Design review of the part shown in the three views and the two pictorial views. Dimensions are in mm from the part's minimum x, y and z. A direction names the side the tool comes from. Round coordinates to 2 decimals unless told otherwise and drop trailing zeros. Order: outer loops, then holes, each group sorted by start corner. A loop starts at its lowest first (then second) coordinate and runs counter-clockwise, first axis right, second up. Notation, with made-up numbers: M -4,61 L 3,61 A23 cw 3,81 Z; hole C 81.5,3.5 d4. An arc over 180 degrees is marked long. Use a Markdown table: item, result. Add a question column.
(1) For pin 1 (1 mm diameter, centred on x = 4.5, y = 13, fed in from +Z); pin 2 (4 mm diameter, centred on x = 4.5, z = 20.5, fed in from -Y); pin 3 (4 mm diameter, centred on y = 20.5, z = 34, fed in from +X), all flat-tipped, find the tip position at first contact; note any pin that passes through.
(2) Machinability: for the marked faces 4, 5 and 6, which of the approach directions +Z, -Z, +X, -X, +Y, -Y give a long, thin tool a straight path to every point of the face, cutting with its end or side? Answer none if there is none.
(3) Take a section at C-C (y = 18). Write out the cut boundary in (x, z) (1 decimal).
(4) To check wall thickness, follow probe 1 along Z at (x, y) = (23, 8); probe 2 along Z at (x, y) = (17, 2.5); probe 3 along X at (y, z) = (18.5, 8). State the ranges of each line that lie inside material, in increasing order. Write a range as from..to.
(5) Take a section at B-B (x = 16). Write out the cut boundary in (y, z).
(6) The part is to be moulded in two halves that separate along Y. For the marked faces 1, 2 and 3, say which applies: released by +Y, released by -Y, zero draft, split by the parting line, or undercut.
(7) Take a section at A-A (z = 46.5). Write out the cut boundary in (x, y).
(8) Take a section at D-D (z = 18). Write out the cut boundary in (x, y).
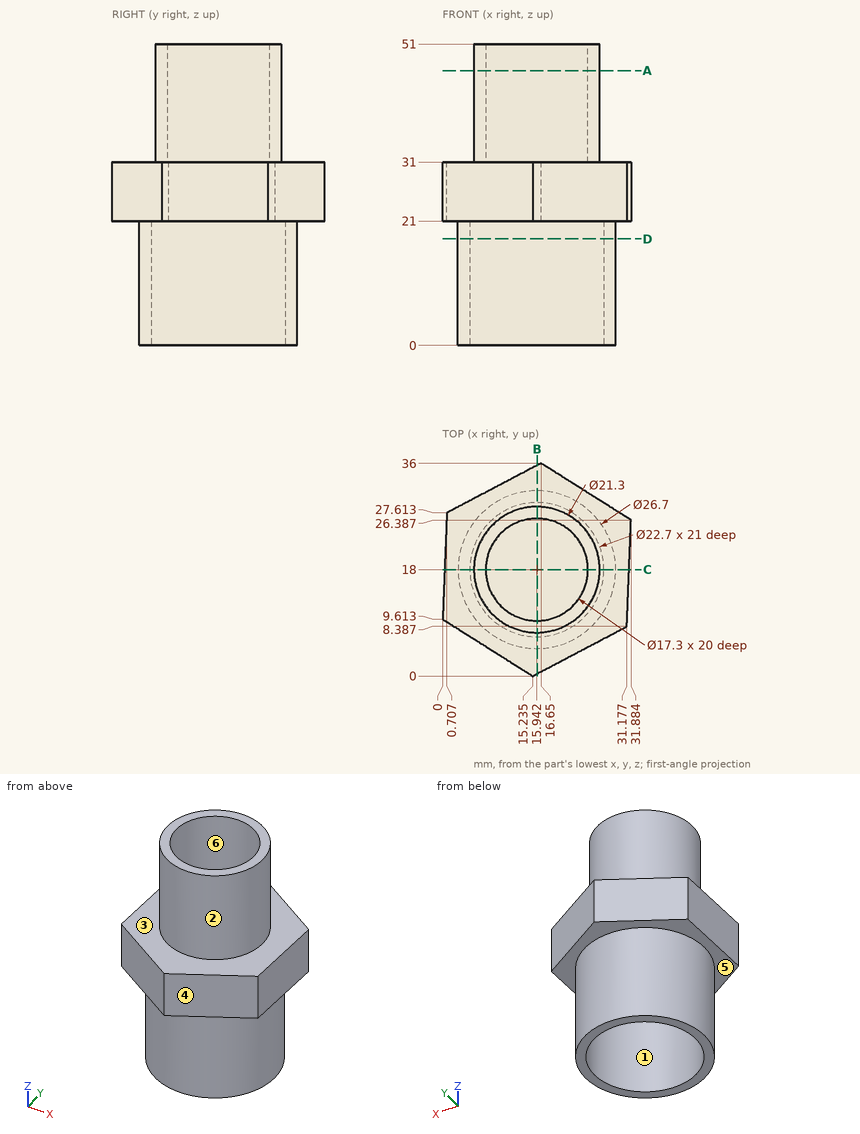
Verdict:
| question | item | result |
|---|---|---|
| 1 | pin 1 | stops at z = 31 |
| 1 | pin 2 | stops at y = 5.55 |
| 1 | pin 3 | stops at x = 26.58 |
| 2 | face 4 | +Z, -Z, +X, -Y |
| 2 | face 5 | -Z |
| 2 | face 6 | +Z |
| 3 | outline | M 0.3,21 L 2.6,21 L 2.6,0 L 4.6,0 L 4.6,21 L 27.3,21 L 27.3,0 L 29.3,0 L 29.3,21 L 31.6,21 L 31.6,31 L 26.6,31 L 26.6,51 L 24.6,51 L 24.6,31 L 7.3,31 L 7.3,51 L 5.3,51 L 5.3,31 L 0.3,31 Z |
| 4 | probe 1 | z = 0..31 |
| 4 | probe 2 | z = 21..31 |
| 4 | probe 3 | x = 2.6..4.6, 27.28..29.28 |
| 5 | outline | M 0.4,21 L 4.65,21 L 4.65,0 L 6.65,0 L 6.65,21 L 29.35,21 L 29.35,0 L 31.35,0 L 31.35,21 L 35.66,21 L 35.66,31 L 28.65,31 L 28.65,51 L 26.65,51 L 26.65,31 L 9.35,31 L 9.35,51 L 7.35,51 L 7.35,31 L 0.4,31 Z |
| 6 | face 1 | undercut |
| 6 | face 2 | split by the parting line |
| 6 | face 3 | zero draft |
| 7 | outline | C 15.94,18 d21.3; hole C 15.94,18 d17.3 |
| 8 | outline | C 15.94,18 d26.7; hole C 15.94,18 d22.7 |
